The model under review builds one solid part; all positions refer to its coordinate system, in mm. A direction names the side the tool comes from. Coordinates: 2 decimals unless noted, no trailing zeros. Order: outer loops, then holes, each group sorted by start corner. A loop starts at its lowest first (then second) coordinate and runs counter-clockwise, first axis right, second up. Notation, with made-up numbers: (-18, -38) -> (24, -38) arc R20 ccw to (24, -10) -> close; hole circle Ø3 at (30, 57). An arc over 180 degrees is marked (long way). Use one line per item in the form item = value.
from build123d import *

# Parameters (mm, degrees)
SKETCH038_W             = 10
SKETCH038_H             = 10
PAD014_DEPTH            = 8
SKETCH039_R             = 1.45
POCKET009_DEPTH         = 5
SKETCH040_W             = 6.2
SKETCH040_H             = 1.8
POCKET010_DEPTH         = 15
BODY014_PLACEMENT_ANGLE = 60


with BuildPart() as part:
    # Sketch038 → Pad014 (new body)
    with BuildSketch(Plane.XY):
        with Locations((0.72243, -0.901424)):
            Rectangle(SKETCH038_W, SKETCH038_H)
    extrude(amount=PAD014_DEPTH)

    # Sketch039 (on Face6 of Pad014) → Pocket009 (cut)
    with BuildSketch(Plane.XY.offset(8)):
        with Locations((0.772802, -1.024983)):
            Circle(SKETCH039_R)
    extrude(amount=-POCKET009_DEPTH, mode=Mode.SUBTRACT)

    # Sketch040 (on Face2 of Pocket009) → Pocket010 (cut)
    with BuildSketch(Plane(origin=(-4.27757, 0, 0), x_dir=(0, -1, 0), z_dir=(-1, 0, 0))):
        with Locations((0.940135, 3.059345)):
            Rectangle(SKETCH040_W, SKETCH040_H)
    extrude(amount=-POCKET010_DEPTH, mode=Mode.SUBTRACT)


with BuildPart() as part_1:
    # Body014 placement: moved
    add(part.part.moved(Location((43.303848, 29, 26.401924))).rotate(Axis((43.303848, 29, 26.401924), (0, 1, 0)), BODY014_PLACEMENT_ANGLE))


solid = part_1.part
Item 1: To check wall thickness, follow L1, parallel to Y at x = 44.75, z = 29.5; L2, parallel to X at y = 27, z = 25; L3, parallel to X at y = 28.25, z = 23.5. State the ranges of each line that lie inside material, in increasing order. Write a range as from..to.
Results found:
L1 = 23.1..24.96, 31.16..33.1
L2 = 44.11..46.61, 48.69..52.32
L3 = 44.98..47.47, 49.55..49.72
Item 2: Tool access review of faces 1 (the face through (45.35, 28.029, 32.523)), 2 (the face through (46, 24.96, 27)): name each direction out of +Z, -Z, +X, -X, +Y, -Y from which nothing blocks a thin tool from reaching the whole face with its end or side.
Results found:
face_1 = +Z, -X, +Y, -Y
face_2 = none
Item 3: We need section C-C (x = 43.25). Write out the cut boundary in (y, z), plus the area to 3 significant figures.
Results found:
outline = (23.1, 26.5) -> (33.1, 26.5) -> (33.1, 31.31) -> (31.16, 31.31) -> (31.16, 30.81) -> (24.96, 30.81) -> (24.96, 31.31) -> (23.1, 31.31) -> close
area = 45.1 mm²
Item 4: Clearance check with flat-ended pins moving along their axes: pin 1 (1.5 mm diameter, centred on x = 46.5, y = 28, fed in from +Z); pin 2 (1 mm diameter, centred on y = 26.5, z = 31, fed in from -X); pin 3 (1 mm diameter, centred on x = 45, y = 30, fed in from +Z); pin 4 (4 mm diameter, centred on x = 46.5, y = 24.5, fed in from -Z). State where each tip first meets the part, or that it passes through.
Results found:
pin_1 = 33.62
pin_2 = 41.85
pin_3 = 32.61
pin_4 = 21.45
Item 5: We need section B-B (x = 45.75). Write out the cut boundary in (y, z).
Results found:
outline = (23.1, 22.17) -> (33.1, 22.17) -> (33.1, 32.75) -> (23.1, 32.75) -> close; hole (24.96, 26.48) -> (31.16, 26.48) -> (31.16, 30.08) -> (24.96, 30.08) -> close
Item 6: We need section A-A (y = 31.75). Write out the cut boundary in (x, z).
Results found:
outline = (41.17, 30.11) -> (46.17, 21.45) -> (53.09, 25.45) -> (48.09, 34.11) -> close
Item 7: Draft analysis for pull direction Y (two halves, no side actions). For faces 3 (the face through (47, 33.099, 28)), 4 (the face through (46, 31.16, 27)), 5 (the face through (50, 29.3, 30.8)), 6 (the face through (47, 23.099, 28)), state which applies: released by +Y, released by -Y, zero draft, split by the parting line, or undercut.
Results found:
face_3 = released by +Y
face_4 = undercut
face_5 = zero draft
face_6 = released by -Y
Item 8: We need section D-D (z = 32.75). Write out the cut boundary in (x, y), plus the area to 3 significant figures.
Results found:
outline = (45.74, 23.1) -> (48.88, 23.1) -> (48.88, 33.1) -> (45.74, 33.1) -> close
area = 31.3 mm²
